Autodesk Inventor part; units mm, degrees
ref_plane "YZ Plane" through (0, 0, 0) normal (1, 0, 0) x (0, 1, 0)
ref_plane "XZ Plane" through (0, 0, 0) normal (0, 1, 0) x (-1, 0, 0)
ref_plane "XY Plane" through (0, 0, 0) normal (0, 0, 1) x (1, 0, 0)
sketch "Эскиз1" plane through (0, 0, 0) normal (0, 0, 1) x (1, 0, 0)
  line L0 (-26.3955, 0) -> (-26.3955, 30)
  line L1 (228.6045, 0) -> (228.6045, 60.0004)
  circle A0 centre (221.1045, 7.5) radius 2
  circle A1 centre (-18.8955, 7.5) radius 2
  line L2 (-26.3955, 60.0004) -> (-30.3955, 60.0004)
  line L3 (-26.3955, 60.0004) -> (228.6045, 60.0004)
  line L4 (228.6045, 0) -> (-26.3955, 0)
  line L5 (-26.3955, 0) -> (-26.3955, 60.0004)
  point P0 (0, 0)
  dimension "d19" = 7.5
  dimension "d20" = 7.5
  dimension "d21" = 255
extrude "Выдавливание1" add sketch "Эскиз1" along normal blind 4
thicken "Толщина1" operation add thickness 4 both sides no extend neighbours yes toward (1, 0, 0) faces at (228.6045, 20.0001, 2.6667)
thicken "Толщина2" operation add thickness 4 both sides no extend neighbours yes toward (-1, 0, 0) faces at (-26.3955, 40.0003, 2.6667)
sketch "Эскиз2" plane through (0, 0, 4) normal (0, 0, 1) x (1, 0, 0)
  line L0 (232.6045, 60.0004) -> (-30.3955, 60.0004)
  line L1 (-30.3955, 60.0004) -> (-26.3955, 60.0004)
  line L2 (-26.3955, 60.0004) -> (-26.3955, 48.0004)
  line L3 (-26.3955, 48.0004) -> (-30.3955, 48.0004)
  line L4 (-30.3955, 48.0004) -> (-30.3955, 60.0004)
  line L5 (232.6045, 60.0004) -> (228.6045, 60.0004)
  line L6 (228.6045, 60.0004) -> (228.6045, 48.0004)
  line L7 (228.6045, 48.0004) -> (232.6045, 48.0004)
  line L8 (232.6045, 48.0004) -> (232.6045, 60.0004)
  point P0 (0, 0)
  point P1 (228.6045, 60.0004)
  dimension "d6" = 4
  dimension "d7" = 12
  dimension "d8" = 4
  dimension "d9" = 12
extrude "Выдавливание2" cut sketch "Эскиз2" against normal blind 4
pattern_linear "Прямоуг.массив1" count 3 spacing 24 along (0, -1, 0) of "Выдавливание2"
thicken "Толщина3" operation add thickness 4 both sides no extend neighbours yes toward (1, 0, 0) faces at (-30.3955, 0.0003, 1.3333) (-29.0622, 0.0004, 2.6667)
thicken "Толщина4" operation add thickness 4 both sides no extend neighbours yes toward (-1, 0, 0) faces at (232.6045, 0.0001, 1.3333) (229.9378, 0.0004, 2.6667)
properties part number "KB33-046-004-014 - Лицевая вертикальня пластина" material "Пластик ПЭТ"
Geometry check sheet. Reference: the model listing, model coordinates, mm. Give positions to 0.01 mm unless a question says otherwise; leave off trailing zeros. Order: outer loops, then holes, each group sorted by start corner. A loop starts at its lowest first (then second) coordinate and runs counter-clockwise, first axis right, second up.
1. Thickness scan on L1, parallel to X at y = 7.5, z = 1.5; L2, parallel to X at y = 3, z = 2.2. Record the ranges inside material, lowest first.
2. Gauge pin test, flat ends, axial feed: pin 1 Ø1.5 at (y, z) = (52, 2) entering from +X; pin 2 Ø1.2 at (x, z) = (-27.5, 2) entering from +Y; pin 3 Ø1.2 at (x, z) = (-27.5, 2.5) entering from -Y. Record the tip position at first contact, or that the pin passes through.
3. Section check B-B, the plane y = 55. Enter the section's corners in (x, z).
4. Section check A-A, the plane z = 3.05. Enter the section's corners in (x, y), and give its area (3 significant figures).
Values follow:
1. L1: x = -26.4 to -20.9, -16.9 to 219.1, 223.1 to 228.6
1. L2: x = -26.4 to 228.6
2. pin 1: stops at x = 228.6
2. pin 2: stops at y = 48
2. pin 3: stops at y = 12
3. outline: (-26.4, 0) - (228.6, 0) - (228.6, 4) - (-26.4, 4) - close
4. outline: (-30.4, 12) - (-26.4, 12) - (-26.4, 0) - (228.6, 0) - (228.6, 12) - (232.6, 12) - (232.6, 24) - (228.6, 24) - (228.6, 36) - (232.6, 36) - (232.6, 48) - (228.6, 48) - (228.6, 60) - (-26.4, 60) - (-26.4, 48) - (-30.4, 48) - (-30.4, 36) - (-26.4, 36) - (-26.4, 24) - (-30.4, 24) - close; hole circle Ø4 at (-18.9, 7.5); hole circle Ø4 at (221.1, 7.5)
4. area: 15,500 mm2
